For this review, take the finished solid that the model builds, in its own axes (mm). A direction names the side the tool comes from. Give positions to 0.01 mm unless a question says otherwise; leave off trailing zeros. Loops run counter-clockwise (first coordinate to the right, second up) from the corner with the lowest first, then second, coordinate; pieces in that order, holes last. Notation, with made-up numbers: (70, 51) - (74, 51) arc R20 ccw to (74, 82) - close; hole circle Ø11 at (-12.75, -9). An arc over 180 degrees is marked (long way). Answer as CSV lines item,"result".
Autodesk Inventor part; units mm, degrees
ref_plane "YZ Plane" through (0, 0, 0) normal (1, 0, 0) x (0, 1, 0)
ref_plane "XZ Plane" through (0, 0, 0) normal (0, 1, 0) x (-1, 0, 0)
ref_plane "XY Plane" through (0, 0, 0) normal (0, 0, 1) x (1, 0, 0)
sketch "Esquisse1" plane through (0, 0, 0) normal (0, 0, 1) x (1, 0, 0)
  line L0 (-1, -22.45) -> (1, -22.45)
  line L1 (-1, -21.45) -> (-1, -22.45)
  line L2 (-3, -21.45) -> (-1, -21.45)
  line L3 (-3, -21.45) -> (-3, -34.3)
  line L4 (-3, -34.3) -> (-13.5643, -34.3)
  line L5 (-13.5643, -34.3) -> (-13.5643, 34.3)
  line L6 (-13.5643, 34.3) -> (-3, 34.3)
  line L7 (-3, 21.45) -> (-3, 34.3)
  line L8 (-1, 21.45) -> (-3, 21.45)
  line L9 (-1, 22.45) -> (-1, 21.45)
  line L10 (1, 22.45) -> (-1, 22.45)
  line L11 (1, 21.45) -> (1, 22.45)
  line L12 (3, 21.45) -> (1, 21.45)
  line L13 (3, 24.45) -> (3, 21.45)
  line L14 (3, 24.45) -> (3.0074, 24.45)
  line L15 (3.0074, 24.45) -> (3.0074, 34.3)
  line L16 (3.0074, 34.3) -> (15.5357, 34.3)
  line L17 (15.5357, 34.3) -> (15.5357, 30.7219)
  line L18 (15.5357, 30.7219) -> (17.5357, 30.7219)
  line L19 (17.5357, 30.7219) -> (17.5357, 34.3)
  line L20 (17.5357, 34.3) -> (21.4357, 34.3)
  line L21 (21.4357, 34.3) -> (21.4357, 30.7219)
  line L22 (21.4357, 30.7219) -> (23.4357, 30.7219)
  line L23 (23.4357, 30.7219) -> (23.4357, 36.3)
  line L24 (-16.5643, 36.3) -> (23.4357, 36.3)
  line L25 (-16.5643, 36.3) -> (-16.5643, -36.3)
  line L26 (-16.5643, -36.3) -> (23.4357, -36.3)
  line L27 (23.4357, -30.7219) -> (23.4357, -36.3)
  line L28 (23.4357, -30.7219) -> (21.4357, -30.7219)
  line L29 (21.4357, -30.7219) -> (21.4357, -34.3)
  line L30 (21.4357, -34.3) -> (17.5357, -34.3)
  line L31 (17.5357, -34.3) -> (17.5357, -30.7219)
  line L32 (17.5357, -30.7219) -> (15.5357, -30.7219)
  line L33 (15.5357, -30.7219) -> (15.5357, -34.3)
  line L34 (15.5357, -34.3) -> (3.0074, -34.3)
  line L35 (3.0074, -34.3) -> (3.0074, -24.45)
  line L36 (3.0074, -24.45) -> (3, -24.45)
  line L37 (3, -21.45) -> (3, -24.45)
  line L38 (1, -21.45) -> (3, -21.45)
  line L39 (1, -22.45) -> (1, -21.45)
  line L40 (23.4357, 36.3) -> (-16.5643, 36.3)
  line L41 (-16.5643, 36.3) -> (-16.5643, -36.3)
  line L42 (-16.5643, -36.3) -> (23.4357, -36.3)
  line L43 (23.4357, -36.3) -> (23.4357, 36.3)
  line L44 (-18.5643, 38.3) -> (25.4357, 38.3)
  line L45 (25.4357, 38.3) -> (25.4357, -38.3)
  line L46 (25.4357, -38.3) -> (-18.5643, -38.3)
  line L47 (-18.5643, -38.3) -> (-18.5643, 38.3)
  point P0 (0, 0)
  dimension "d0" = 2
extrude "Extrusion1" add sketch "Esquisse1" along normal blind 2 contours L1 L2 L3 L4 L5 L6 L7 L8 L9 L10 L11 L12 L13 L14 L15 L16 L17 L18 L19 L20 L21 L22 L43 L28 L29 L30 L31 L32 L33 L34 L35 L36 L37 L38 L39 L0 | L0 L39 L38 L37 L36 L35 L34 L33 L32 L31 L30 L29 L28 L27 L26 L25 L24 L23 L22 L21 L20 L19 L18 L17 L16 L15 L14 L13 L12 L11 L10 L9 L8 L7 L6 L5 L4 L3 L2 L1 | L44 L45 L46 L47
sketch "Esquisse2" plane through (0, 0, 0) normal (0, 0, -1) x (-1, 0, 0)
  line L0 (-23.4357, -36.3) -> (-23.4357, 36.3)
  line L1 (16.5643, 36.3) -> (-23.4357, 36.3)
  line L2 (16.5643, 36.3) -> (16.5643, -36.3)
  line L3 (16.5643, -36.3) -> (-23.4357, -36.3)
  line L4 (18.5643, -38.3) -> (-25.4357, -38.3)
  line L5 (18.5643, 38.3) -> (18.5643, -38.3)
  line L6 (-25.4357, 38.3) -> (18.5643, 38.3)
  line L7 (-25.4357, -38.3) -> (-25.4357, 38.3)
  point P0 (0, 0)
extrude "Extrusion2" add sketch "Esquisse2" along normal blind 2
sketch "Esquisse3" plane through (0, 0, -2) normal (0, 0, -1) x (-1, 0, 0)
  line L0 (-23.4357, -36.3) -> (16.5643, -36.3) construction
  line L1 (16.5643, 36.3) -> (-23.4357, 36.3) construction
  line L2 (16.5643, -36.3) -> (-23.4357, 36.3) construction
  line L3 (-23.4357, -36.3) -> (16.5643, 36.3) construction
  line L4 (-23.9357, 36.7319) -> (17.0643, 36.7319)
  line L5 (17.0643, 36.7319) -> (17.0643, -36.7319)
  line L6 (17.0643, -36.7319) -> (-23.9357, -36.7319)
  line L7 (-23.9357, -36.7319) -> (-23.9357, 36.7319)
  line L8 (-23.9357, 36.7319) -> (17.0643, -36.7319) construction
  line L9 (17.0643, 36.7319) -> (-23.9357, -36.7319) construction
  line L10 (16.5643, 36.3) -> (16.5643, -36.3)
  point P0 (0, 0)
  point P1 (-3.4357, 0)
  dimension "d5" = 0.5
extrude "Extrusion3" cut sketch "Esquisse3" against normal blind 2
properties part number "Cache_remote"
1) Wall thickness on line 1 (X direction, y = 33, z = -0.4); line 2 (Y direction, x = 4.5, z = -0.2); line 3 (Z direction, x = -4.5, y = -10): over which ranges is each line inside the solid? List them lowest first. Write a range as from..to.
From the geometry:
line 1,"x = -18.56..-17.06, 23.94..25.44"
line 2,"y = -38.3..-36.73, 36.73..38.3"
line 3,"z = 0..2"
2) Insertion check: P1, Ø12.5, axis at x = 5.5, y = -10, coming from the -Z side. The pin has a flat end and moves straight along its axis. Give the tip position at first contact, or say it passes through.
From the geometry:
P1,"stops at z = 0"
3) Consider section B-B on y = 21.5. Write out the cut boundary in (x, z).
From the geometry:
outline,"(-18.56, -2) - (-17.06, -2) - (-17.06, 0) - (23.94, 0) - (23.94, -2) - (25.44, -2) - (25.44, 2) - (-18.56, 2) - close"
4) Consider section C-C on x = 5.5. Write out the cut boundary in (y, z).
From the geometry:
outline,"(-38.3, -2) - (-36.73, -2) - (-36.73, 0) - (36.73, 0) - (36.73, -2) - (38.3, -2) - (38.3, 2) - (-38.3, 2) - close"
5) Machinability: for faces 1 (the flat face through (3, -36.732, -1)), 2 (the flat face through (3, 1, 2)), which of the approach directions +Z, -Z, +X, -X, +Y, -Y give a long, thin tool a straight path to every point of the face, cutting with its end or side? Answer none if there is none.
From the geometry:
face 1,"-Z"
face 2,"+Z, +X, -X, +Y, -Y"
6) Draft analysis for pull direction Y (two halves, no side actions). For faces 3 (the flat face through (4, 38.3, 0)), 4 (the flat face through (25.436, -1, 0)), 5 (the flat face through (-17.064, 1, -1)), 6 (the flat face through (23.936, -1, -1)), state which applies: pulls with the +Y half, pulls with the -Y half, needs draft (parallel to the pull), parting line crosses it, or undercut.
From the geometry:
face 3,"pulls with the +Y half"
face 4,"needs draft"
face 5,"undercut"
face 6,"undercut"
7) Consider section A-A on z = -0.95. Write out the cut boundary in (x, y).
From the geometry:
outline,"(-18.56, -38.3) - (25.44, -38.3) - (25.44, 38.3) - (-18.56, 38.3) - close; hole (-17.06, -36.73) - (23.94, -36.73) - (23.94, 36.73) - (-17.06, 36.73) - close"
